Work out the finished part from the listing and answer in its coordinate system (mm). A direction names the side the tool comes from. Give positions to 0.01 mm unless a question says otherwise; leave off trailing zeros. Loops run counter-clockwise (first coordinate to the right, second up) from the corner with the lowest first, then second, coordinate; pieces in that order, holes last.
```python
from build123d import *

# Parameters (mm, degrees)
PAD029_DEPTH            = 5.5
SKETCH060_R             = 3.9
PAD030_DEPTH            = 25
CHAMFER011_SIZE         = 1
CHAMFER012_SIZE         = 0.5
BODY020_PLACEMENT_ANGLE = 180


with BuildPart() as part:
    # Sketch059 → Pad029 (new body)
    with BuildSketch(Plane.XY):
        Polygon((7.25, 0), (3.625, 6.278684), (-3.625, 6.278684), (-7.25, 0), (-3.625, -6.278684), (3.625, -6.278684), align=None)
    extrude(amount=PAD029_DEPTH)

    # Sketch060 (on Face7 of Pad029) → Pad030 (join)
    with BuildSketch(Plane(origin=(0, 0, 0), x_dir=(1, 0, 0), z_dir=(0, 0, -1))):
        Circle(SKETCH060_R)
    extrude(amount=PAD030_DEPTH)

    # Chamfer011
    chamfer011_edges = [part.edges().sort_by_distance(p)[0] for p in [
        (-3.9, 0, -25),
    ]]
    chamfer(chamfer011_edges, length=CHAMFER011_SIZE)

    # Chamfer012
    chamfer012_edges = [part.edges().sort_by_distance(p)[0] for p in [
        (5.4375, 3.139342, 5.5),
        (0, 6.278684, 5.5),
        (-5.4375, 3.139342, 5.5),
        (-5.4375, -3.139342, 5.5),
        (0, -6.278684, 5.5),
        (5.4375, -3.139342, 5.5),
    ]]
    chamfer(chamfer012_edges, length=CHAMFER012_SIZE)


with BuildPart() as part_1:
    # Body020 placement: moved
    add(part.part.moved(Location((0, 0, 284))).rotate(Axis((0, 0, 284), (1, 0, 0)), BODY020_PLACEMENT_ANGLE))


solid = part_1.part
```
Q1. Section C-C on z = 297.5 is taken. Give the vertices of the cut face in (x, y), plus the area to 3 significant figures.
Q2. Which of the six approach directions +Z, -Z, +X, -X, +Y, -Y give full straight-line access (tool end or side, diameter ignored) to faces 1 (the face through (-3.095, -2.373, 295.832)), 2 (the face through (5.46, -3.1, 281.54))?
Q3. Section A-A on x = 0 is taken. Give the vertices of the cut face in (y, z).
Q4. Section B-B on y = -4.75 is taken. Give the vertices of the cut face in (x, z), plus the area to 3 significant figures.
Q5. Given pin 1 (5 mm diameter, centred on y = 1, z = 287, fed in from -X); pin 2 (6 mm diameter, centred on y = -3, z = 289.5, fed in from +X); pin 3 (4 mm diameter, centred on y = -2.5, z = 283, fed in from +X), each flat-ended and moving along its own axis, determine where each tip first touches the part or whether it passes through.
Q6. Section D-D on x = 5.75 is taken. Give the vertices of the cut face in (y, z), plus the area to 3 significant figures.
Q7. Consider line 1 along Z through (x, y) = (3, 4); line 2 along Z through (x, y) = (-2, -2.5); line 3 along X through (y, z) = (3.5, 283). Determine where each line is inside the solid, lowest interval first.
Check result:
1. outline: circle Ø7.8 at (0, 0)
1. area: 47.8 mm2
2. face 1: +Z
2. face 2: +Z, -Z, +X, -Y
3. outline: (-6.28, 279) - (-5.78, 278.5) - (5.78, 278.5) - (6.28, 279) - (6.28, 284) - (3.9, 284) - (3.9, 308) - (2.9, 309) - (-2.9, 309) - (-3.9, 308) - (-3.9, 284) - (-6.28, 284) - close
4. outline: (-4.51, 279) - (-3.93, 278.5) - (3.93, 278.5) - (4.51, 279) - (4.51, 284) - (-4.51, 284) - close
4. area: 49.3 mm2
5. pin 1: stops at x = -3.9
5. pin 2: stops at x = 3.9
5. pin 3: stops at x = 6.96
6. outline: (-2.6, 279) - (-1.6, 278.5) - (1.6, 278.5) - (2.6, 279) - (2.6, 284) - (-2.6, 284) - close
6. area: 28.1 mm2
7. line 1: z = 278.5 to 284
7. line 2: z = 278.5 to 308.7
7. line 3: x = -5.23 to 5.23
